For this review, use the dimensioned drawing (mm, ordinates from the lowest corner) and the shaded views. A direction names the side the tool comes from. Round coordinates to 2 decimals unless told otherwise and drop trailing zeros. Order: outer loops, then holes, each group sorted by start corner. A loop starts at its lowest first (then second) coordinate and runs counter-clockwise, first axis right, second up. Notation, with made-up numbers: M 88.5,-8 L 106.5,-8 A24 ccw 106.5,23 Z; hole C -12,-1 d1. An arc over 180 degrees is marked long. One line per item, written item: value. Start each with the question number.
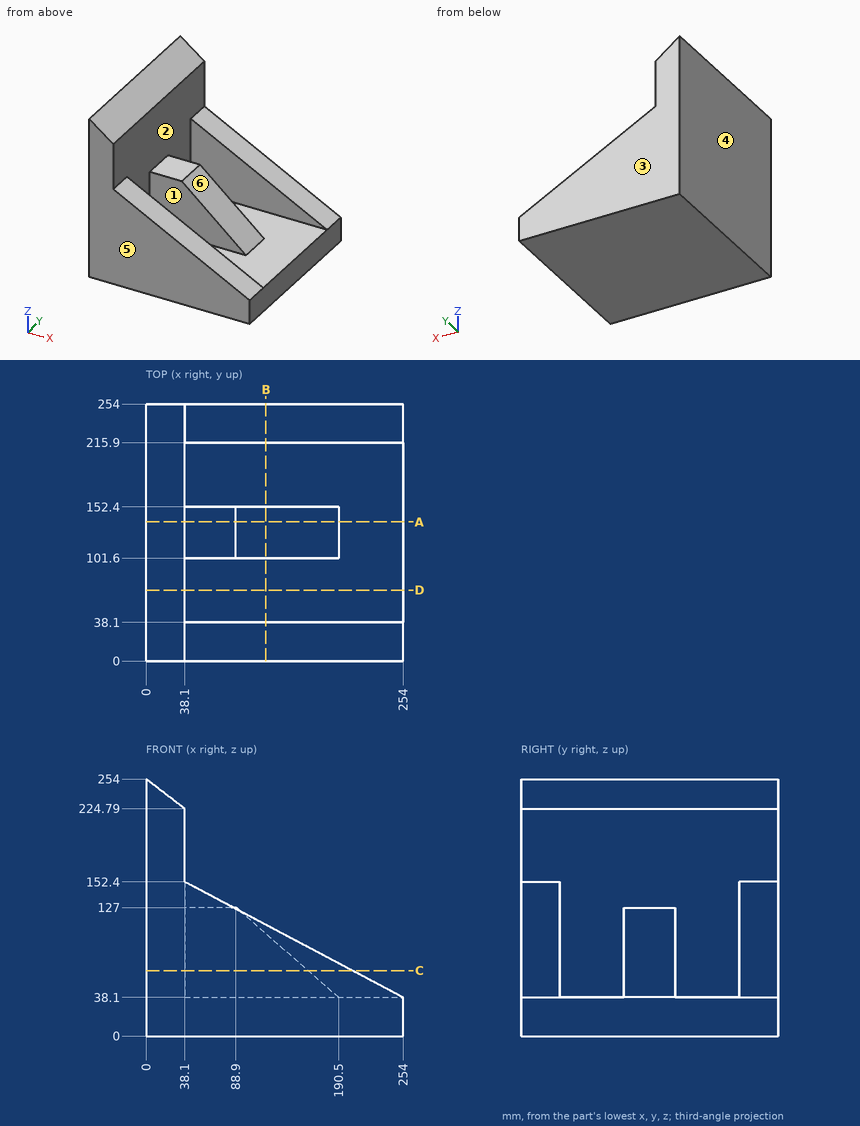
Item 1: Consider section A-A, the plane y = 137.5. Give the boundary of the cut face in (x, z), then the cut area to 3 significant figures.
Item 2: Consider section B-B, the plane x = 118.5. Give the boundary of the cut face in (y, z).
Item 3: The part is to be moulded in two halves that separate along Y. For the marked faces 1, 2, 3 and 4, say which applies: pulls with the +Y half, pulls with the -Y half, needs draft (parallel to the pull), parting line crosses it, or undercut.
Item 4: Wall thickness on L1, parallel to Y at x = 103, z = 76; L2, parallel to Y at x = 116, z = 105.5; L3, parallel to X at y = 91, z = 86: over which ranges is each line inside the solid? List them lowest first.
Item 5: Consider section C-C, the plane z = 64.5. Give the boundary of the cut face in (x, y), then the cut area to 3 significant figures.
Item 6: Clearance check with flat-ended pins moving along their axes: P1, Ø1, axis at y = 207.5, z = 220.5, coming from the +X side; P2, Ø1.5, axis at x = 185.5, y = 147.5, coming from the +Z side; P3, Ø2, axis at x = 33.5, y = 175.5, coming from the +Z side. State where each tip first meets the part, or that it passes through.
Item 7: Machinability: for the marked faces 5 and 6, which of the approach directions +Z, -Z, +X, -X, +Y, -Y give a long, thin tool a straight path to every point of the face, cutting with its end or side? Answer none if there is none.
Item 8: Consider section D-D, the plane y = 70. Give the boundary of the cut face in (x, z), then the cut area to 3 significant figures.
Computed:
1. outline: M 0,0 L 254,0 L 254,38.1 L 190.5,38.1 L 88.9,127 L 38.1,127 L 38.1,224.79 L 0,254 Z
1. area: 26,400 mm^2
2. outline: M 0,0 L 254,0 L 254,109.84 L 215.9,109.84 L 215.9,38.1 L 152.4,38.1 L 152.4,101.1 L 101.6,101.1 L 101.6,38.1 L 38.1,38.1 L 38.1,109.84 L 0,109.84 Z
3. face 1: undercut
3. face 2: undercut
3. face 3: pulls with the +Y half
3. face 4: needs draft
4. L1: y = 0 to 38.1, 101.6 to 152.4, 215.9 to 254
4. L2: y = 0 to 38.1, 215.9 to 254
4. L3: x = 0 to 38.1
5. outline: M 0,0 L 204.13,0 L 204.13,38.1 L 38.1,38.1 L 38.1,101.6 L 160.33,101.6 L 160.33,152.4 L 38.1,152.4 L 38.1,215.9 L 204.13,215.9 L 204.13,254 L 0,254 Z
5. area: 28,500 mm^2
6. P1: stops at x = 38.1
6. P2: stops at z = 43.13
6. P3: stops at z = 229.08
7. face 5: +Z, -Z, +X, -X, -Y
7. face 6: +Z, +X
8. outline: M 0,0 L 254,0 L 254,38.1 L 38.1,38.1 L 38.1,224.79 L 0,254 Z
8. area: 17,300 mm^2
